```python
from build123d import *

# Parameters (mm, degrees)
SKETCH1_R           = 40
BOSS_EXTRUDE1_DEPTH = 3
SKETCH2_R           = 2.5
BOSS_EXTRUDE2_DEPTH = 4


with BuildPart() as part:
    # Sketch1 → Boss-Extrude1 (new body)
    with BuildSketch(Plane(origin=(0, 0, 0), x_dir=(1, 0, 0), z_dir=(0, 1, 0))):
        with Locations(Location((0, 0, 0), (0, 0, 270))):
            Circle(SKETCH1_R)
    extrude(amount=BOSS_EXTRUDE1_DEPTH)

    # Sketch2 → Boss-Extrude2 (add)
    with BuildSketch(Plane(origin=(0, 3, 0), x_dir=(1, 0, 0), z_dir=(0, 1, 0))):
        with Locations(Location((0, 30, 0), (0, 0, 270))):
            Circle(SKETCH2_R)
        with Locations(Location((21.213203436, 21.213203436, 0), (0, 0, 270))):
            Circle(SKETCH2_R)
        with Locations(Location((30, 0, 0), (0, 0, 270))):
            Circle(SKETCH2_R)
        with Locations(Location((21.213203436, -21.213203436, 0), (0, 0, 270))):
            Circle(SKETCH2_R)
        with Locations(Location((0, -30, 0), (0, 0, 270))):
            Circle(SKETCH2_R)
        with Locations(Location((-21.213203436, -21.213203436, 0), (0, 0, 270))):
            Circle(SKETCH2_R)
        with Locations(Location((-30, 0, 0), (0, 0, 270))):
            Circle(SKETCH2_R)
        with Locations(Location((-21.213203436, 21.213203436, 0), (0, 0, 270))):
            Circle(SKETCH2_R)
    extrude(amount=BOSS_EXTRUDE2_DEPTH)


solid = part.part
```
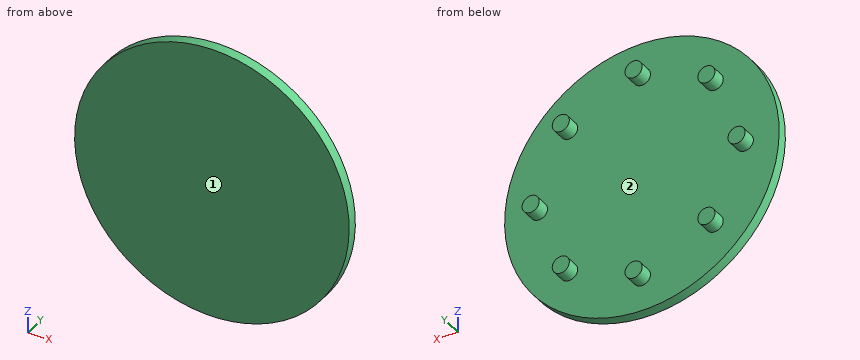
CAD build for the part. Positions are in the model's coordinates, mm. Face numbers are marked on the shaded views. A direction names the side the tool comes from. Round coordinates to 2 decimals unless told otherwise and drop trailing zeros. Order: outer loops, then holes, each group sorted by start corner. A loop starts at its lowest first (then second) coordinate and runs counter-clockwise, first axis right, second up. Notation, with made-up numbers: (-9, 1) - (31, 1) arc R24 cw to (31, 34) - close; hole circle Ø11 at (-33.5, 0). An arc over 180 degrees is marked (long way). Answer in a Markdown table with one row per item. Add a question column.
(1) Band-saw the part on C-C on x = -30. List the corners of the cut face in (y, z).
(2) 3-axis set-ups, long thin cutter, end or side, ignore diameter. For the marked faces 1 and 2: which of +Z, -Z, +X, -X, +Y, -Y reach the whole face in a straight line?
(3) Band-saw the part on B-B on z = 0. List the corners of the cut face in (x, y), and give its area (3 significant figures).
(4) Drop flat-ended pins along their axis: pin 1 Ø3 at (x, z) = (21, 15) entering from +Y; pin 2 Ø2 at (x, y) = (29.5, 5) entering from +Z; pin 3 Ø4 at (y, z) = (4, 29) entering from -X. Give the stop position or say it passes through.
(5) Band-saw the part on D-D on y = 1. List the corners of the cut face in (x, z).
(6) Band-saw the part on A-A on y = 5.25. List the corners of the cut face in (x, z).
(7) Probe L1, parallel to Y at x = 17, z = -13; L2, parallel to X at y = 5.5, z = -21; L3, parallel to X at y = 2, z = -0.5. List the from-to ranges inside material, lowest first. Write a range as [from, to].
Data:
| question | item | result |
|---|---|---|
| 1 | outline | (0, -26.46) - (3, -26.46) - (3, -2.5) - (7, -2.5) - (7, 2.5) - (3, 2.5) - (3, 26.46) - (0, 26.46) - close |
| 2 | face 1 | +Z, -Z, +X, -X, -Y |
| 2 | face 2 | +Y |
| 3 | outline | (-40, 0) - (40, 0) - (40, 3) - (32.5, 3) - (32.5, 7) - (27.5, 7) - (27.5, 3) - (-27.5, 3) - (-27.5, 7) - (-32.5, 7) - (-32.5, 3) - (-40, 3) - close |
| 3 | area | 280 mm^2 |
| 4 | pin 1 | stops at y = 3 |
| 4 | pin 2 | stops at z = 2.5 |
| 4 | pin 3 | stops at x = -29.27 |
| 5 | outline | circle Ø80 at (0, 0) |
| 6 | outline | circle Ø5 at (-30, 0); circle Ø5 at (-21.21, -21.21); circle Ø5 at (-21.21, 21.21); circle Ø5 at (0, -30); circle Ø5 at (0, 30); circle Ø5 at (21.21, -21.21); circle Ø5 at (21.21, 21.21); circle Ø5 at (30, 0) |
| 7 | L1 | y = [0, 3] |
| 7 | L2 | x = [-23.7, -18.72], [18.72, 23.7] |
| 7 | L3 | x = [-40, 40] |
